Build history of the part. All positions in model axes, mm. A direction names the side the tool comes from. Coordinates: 2 decimals unless noted, no trailing zeros. Order: outer loops, then holes, each group sorted by start corner. A loop starts at its lowest first (then second) coordinate and runs counter-clockwise, first axis right, second up. Notation, with made-up numbers: M 0.5,18 L 27.5,18 A19 ccw 27.5,43 Z; hole C 30.25,85 d3. An arc over 180 degrees is marked long. Write item = value, one per line. Start each with the question number.
Q1. Band-saw the part on D-D on y = -93.5. Write the cut outline in (x, z).
Q2. Band-saw the part on B-B on x = 204.5. Write the cut outline in (y, z) (3 decimals), plus the area to 3 significant figures.
Q3. Band-saw the part on C-C on z = 3. State how many separate pieces and enclosed holes the cut face has, plus the area to 3 significant figures.
Q4. Band-saw the part on A-A on x = 62.23. Write the cut outline in (y, z).
Q5. Pin check, flat tips, straight feed: P1, Ø0.8, axis at y = -34.5, z = 12, coming from the -X side; P2, Ø0.6, axis at x = 24.5, z = 12.5, coming from the -Y side (3 decimals); P3, Ø0.8, axis at x = 23, z = 12.5, coming from the +Y side (3 decimals); P4, Ø0.8, axis at y = -137.5, z = 12.5, coming from the -X side. Stop position of each tip, or through.
Q6. Drill centre lines: probe 1 along Y at (x, z) = (195.58, 4.25); probe 2 along X at (y, z) = (-103, 12.25); probe 3 along X at (y, z) = (-43.5, 5.5). Where is each one in solid material? Low to high.
Q7. Pull direction X, two halves, no side cores. Call faces 1 (the face through (111, -74, 11.938)), 2 (the face through (6.44, -143.6, 5.89)), 3 (the face through (202, -116, 12.7)): released by +X, released by -X, zero draft, split by the parting line, or undercut.
Q8. 3-axis set-ups, long thin cutter, end or side, ignore diameter. For faces 4 (the face through (147.33, -71.44, 6.05)), 5 (the face through (33.861, -133.314, 4.767)): which of +Z, -Z, +X, -X, +Y, -Y reach the whole face in a straight line?
```python
from build123d import *

# Parameters (mm, degrees)
SKETCH3_W                                     = 226.06
SKETCH3_H                                     = 149.86
EXTRUDE2_DEPTH                                = 12.7
SKETCH4_W                                     = 226.06
SKETCH4_H                                     = 149.86
SKETCH4_W_2                                   = 22.225
SKETCH4_H_2                                   = 50.8
EXTRUDE4_DEPTH                                = 0.762
CBORE_FOR_1_4_SOCKET_HEAD_CAP_SCREW1_AT_COUNT = 2
CBORE_FOR_1_4_SOCKET_HEAD_CAP_SCREW1_AT_PITCH = 186.028991356
CBORE_FOR_1_4_SOCKET_HEAD_CAP_SCREW1_2_COUNT  = 2
CBORE_FOR_1_4_SOCKET_HEAD_CAP_SCREW1_2_PITCH  = 166.589197204
CBORE_FOR_1_4_SOCKET_HEAD_CAP_SCREW1_3_COUNT  = 2
CBORE_FOR_1_4_SOCKET_HEAD_CAP_SCREW1_3_PITCH  = 63.5
F_1_1_DIAMETER_HOLE1_D                        = 38.1
F_10_32_TAPPED_HOLE1_D                        = 4.0386
SKETCH19_W                                    = 3.175
SKETCH19_H                                    = 133.35
CUT_EXTRUDE1_DEPTH                            = 0.762
F_1_4_20_TAPPED_HOLE1_D                       = 5.1054
CHAMFER1_SIZE                                 = 12.7
F_13_32_0_40625_DIAMETER_HOLE1_D              = 10.31875


with BuildPart() as part:
    # Sketch3 → Extrude2 (new body)
    with BuildSketch(Plane.XY):
        with Locations((113.03, -74.93)):
            Rectangle(SKETCH3_W, SKETCH3_H)
    extrude(amount=EXTRUDE2_DEPTH)

    # Sketch4 → Extrude4 (cut)
    with BuildSketch(Plane.XY.offset(12.7)):
        with Locations((113.03, -74.93)):
            Rectangle(SKETCH4_W, SKETCH4_H)
        with Locations((30.4927, -33.655)):
            Rectangle(SKETCH4_W_2, SKETCH4_H_2, mode=Mode.SUBTRACT)
        with Locations((30.4927, -116.205)):
            Rectangle(SKETCH4_W_2, SKETCH4_H_2, mode=Mode.SUBTRACT)
        with Locations((195.5673, -116.205)):
            Rectangle(SKETCH4_W_2, SKETCH4_H_2, mode=Mode.SUBTRACT)
        with Locations((195.5673, -33.655)):
            Rectangle(SKETCH4_W_2, SKETCH4_H_2, mode=Mode.SUBTRACT)
    extrude(amount=-EXTRUDE4_DEPTH, mode=Mode.SUBTRACT)

    # Sketch9 → CBORE for 1/4 Socket Head Cap Screw1 (revolve, cut)
    with BuildSketch(Plane(origin=(195.58, -106.68, 0), x_dir=(0, 1, 0), z_dir=(1, 0, 0))):
        Polygon((0, 0), (0, 12.7), (3.57124, 12.7), (3.57124, 9.017), (5.55625, 9.017), (5.55625, 0.635), (6.19125, 0), align=None)
    cbore_for_1_4_socket_head_cap_screw1 = revolve(axis=Axis((195.58, -106.68, -6.35), (0, 0, 1)), mode=Mode.SUBTRACT)

    # CBORE for 1/4 Socket Head Cap Screw1 at: CBORE for 1/4 Socket Head Cap Screw1 ×2
    with Locations(*[Vector(-0.887496077, 0.460815271, 0) * (i * CBORE_FOR_1_4_SOCKET_HEAD_CAP_SCREW1_AT_PITCH) for i in range(1, CBORE_FOR_1_4_SOCKET_HEAD_CAP_SCREW1_AT_COUNT)]):
        add(cbore_for_1_4_socket_head_cap_screw1, mode=Mode.SUBTRACT)

    # CBORE for 1_4 Socket Head Cap Screw1 2: CBORE for 1/4 Socket Head Cap Screw1 ×2
    with Locations(*[Vector(-0.991060662, -0.133412012, 0) * (i * CBORE_FOR_1_4_SOCKET_HEAD_CAP_SCREW1_2_PITCH) for i in range(1, CBORE_FOR_1_4_SOCKET_HEAD_CAP_SCREW1_2_COUNT)]):
        add(cbore_for_1_4_socket_head_cap_screw1, mode=Mode.SUBTRACT)

    # CBORE for 1_4 Socket Head Cap Screw1 3: CBORE for 1/4 Socket Head Cap Screw1 ×2
    with Locations(*[(0, i * CBORE_FOR_1_4_SOCKET_HEAD_CAP_SCREW1_3_PITCH, 0) for i in range(1, CBORE_FOR_1_4_SOCKET_HEAD_CAP_SCREW1_3_COUNT)]):
        add(cbore_for_1_4_socket_head_cap_screw1, mode=Mode.SUBTRACT)

    # 1 (1) Diameter Hole1 (through all)
    with Locations(Plane(origin=(163.83, -24.13, 0), x_dir=(-1, 0, 0), z_dir=(0, 0, -1))):
        with Locations((0, 0), (101.6, 0), (101.6, -101.6), (0, -101.6)):
            Hole(F_1_1_DIAMETER_HOLE1_D / 2)

    # #10-32 Tapped Hole1 (through all)
    with Locations(Plane(origin=(0, 0, 0), x_dir=(-1, 0, 0), z_dir=(0, 0, -1))):
        with Locations((-125.73, -136.8552), (-113.03, -13.0048), (-100.33, -136.8552)):
            Hole(F_10_32_TAPPED_HOLE1_D / 2)

    # Sketch19 → Cut-Extrude1 (cut)
    with BuildSketch(Plane.XY.offset(12.7)):
        with Locations((195.58, -74.93)):
            Rectangle(SKETCH19_W, SKETCH19_H)
        with Locations((30.48, -74.93)):
            Rectangle(SKETCH19_W, SKETCH19_H)
    extrude(amount=-CUT_EXTRUDE1_DEPTH, mode=Mode.SUBTRACT)

    # 1/4-20 Tapped Hole1 (through all)
    with Locations(Plane(origin=(0, 0, 0), x_dir=(-1, 0, 0), z_dir=(0, 0, -1))):
        with Locations((-195.58, -128.905), (-195.58, -20.955), (-30.48, -43.18), (-30.48, -106.68)):
            Hole(F_1_4_20_TAPPED_HOLE1_D / 2)

    # Chamfer1
    chamfer1_edges = [part.edges().sort_by_distance(p)[0] for p in [
        (0, 0, 5.969),
        (226.06, 0, 5.969),
        (226.06, -149.86, 5.969),
        (0, -149.86, 5.969),
    ]]
    chamfer(chamfer1_edges, length=CHAMFER1_SIZE)

    # 13/32 (0.40625) Diameter Hole1 (through all)
    with Locations(Plane(origin=(0, 0, 0), x_dir=(-1, 0, 0), z_dir=(0, 0, -1))):
        with Locations((-74.93, -74.93), (-151.13, -74.93)):
            Hole(F_13_32_0_40625_DIAMETER_HOLE1_D / 2)


solid = part.part
```
Recorded:
q1.outline = M 0,0 L 226.06,0 L 226.06,11.94 L 206.68,11.94 L 206.68,12.7 L 197.17,12.7 L 197.17,11.94 L 193.99,11.94 L 193.99,12.7 L 184.45,12.7 L 184.45,11.94 L 41.61,11.94 L 41.61,12.7 L 32.07,12.7 L 32.07,11.94 L 28.89,11.94 L 28.89,12.7 L 19.38,12.7 L 19.38,11.94 L 0,11.94 Z
q2.outline = M -149.86,0 L 0,0 L 0,11.938 L -8.255,11.938 L -8.255,12.7 L -59.055,12.7 L -59.055,11.938 L -90.805,11.938 L -90.805,12.7 L -141.605,12.7 L -141.605,11.938 L -149.86,11.938 Z
q2.area = 1,870 mm2
q3.separate_pieces = 1
q3.enclosed_holes = 17
q3.area = 28,300 mm2
q4.outline = M -149.86,0 L -144.78,0 L -144.78,11.94 L -149.86,11.94 Z; M -106.68,0 L -43.18,0 L -43.18,11.94 L -106.68,11.94 Z; M -5.08,0 L 0,0 L 0,11.94 L -5.08,11.94 Z
q5.P1 = 0
q5.P2 = -141.605
q5.P3 = -8.255
q5.P4 = 19.38
q6.probe_1 = -149.86 to -131.46, -126.35 to -112.24, -101.12 to -48.74, -37.62 to -23.51, -18.4 to 0
q6.probe_2 = 19.38 to 28.89, 32.07 to 41.61, 184.45 to 193.99, 197.17 to 206.68
q6.probe_3 = 0 to 27.95, 33.01 to 190.03, 201.13 to 226.06
q7.face_1 = undercut
q7.face_2 = released by -X
q7.face_3 = zero draft
q8.face_4 = +Z, -Z
q8.face_5 = -Z
